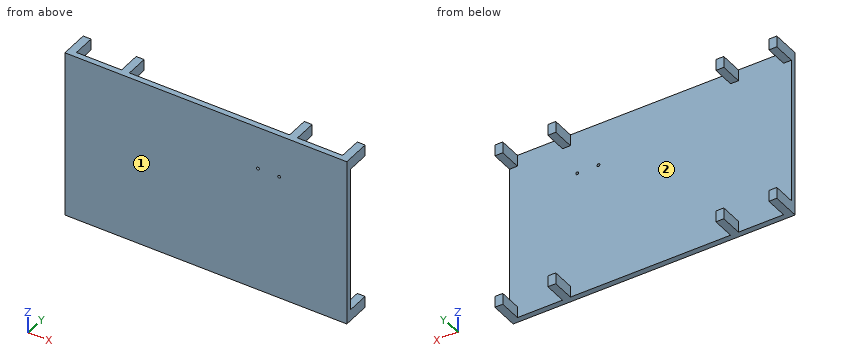
```python
from build123d import *

# Parameters (mm, degrees)
SKETCH1_W           = 250
SKETCH1_H           = 150
BOSS_EXTRUDE1_DEPTH = 5
SKETCH2_W           = 7
SKETCH2_H           = 10
BOSS_EXTRUDE2_DEPTH = 20
SKETCH3_R           = 1.25
CUT_EXTRUDE1_DEPTH  = 148.139389696


with BuildPart() as part:
    # Sketch1 → Boss-Extrude1 (new body)
    with BuildSketch(Plane(origin=(0, 0, 0), x_dir=(1, 0, 0), z_dir=(0, 1, 0))):
        Rectangle(SKETCH1_W, SKETCH1_H)
    extrude(amount=BOSS_EXTRUDE1_DEPTH)

    # Sketch2 → Boss-Extrude2 (add)
    with BuildSketch(Plane(origin=(0, 5, 0), x_dir=(1, 0, 0), z_dir=(0, 1, 0))):
        with Locations((-121.5, -70)):
            Rectangle(SKETCH2_W, SKETCH2_H)
        with Locations((-74.5, -70)):
            Rectangle(SKETCH2_W, SKETCH2_H)
        with Locations((-121.5, 70)):
            Rectangle(SKETCH2_W, SKETCH2_H)
        with Locations((-74.5, 70)):
            Rectangle(SKETCH2_W, SKETCH2_H)
        with Locations((121.5, 70)):
            Rectangle(SKETCH2_W, SKETCH2_H)
        with Locations((74.5, 70)):
            Rectangle(SKETCH2_W, SKETCH2_H)
        with Locations((121.5, -70)):
            Rectangle(SKETCH2_W, SKETCH2_H)
        with Locations((74.5, -70)):
            Rectangle(SKETCH2_W, SKETCH2_H)
    extrude(amount=BOSS_EXTRUDE2_DEPTH)

    # Sketch3 → Cut-Extrude1 (cut, through all)
    with BuildSketch(Plane(origin=(0, 5, 0), x_dir=(1, 0, 0), z_dir=(0, 1, 0))):
        with Locations(Location((46.2, -37, 0), (0, 0, 270))):
            Circle(SKETCH3_R)
        with Locations(Location((65, -37, 0), (0, 0, 270))):
            Circle(SKETCH3_R)
    extrude(amount=-CUT_EXTRUDE1_DEPTH, mode=Mode.SUBTRACT)


solid = part.part
```
Here's how the part is built. I have some questions about the finished solid (model axes, mm). Face numbers are marked on the shaded views. Round coordinates to 2 decimals unless told otherwise and drop trailing zeros. Order: outer loops, then holes, each group sorted by start corner. A loop starts at its lowest first (then second) coordinate and runs counter-clockwise, first axis right, second up. Notation, with made-up numbers: M 68,47 L 92,47 A14 cw 92,65 Z; hole C -4,29 d11. An arc over 180 degrees is marked long. One line per question, with ' | ' between items.
1) I need wall thicknesses on line 1 along X through (y, z) = (16.25, -68); line 2 along X through (y, z) = (3.7, 37); line 3 along Z through (x, y) = (65, 1.8). Which ranges of each line are inside material? Lowest first, please.
Working result:
line 1: -125 to -118, -78 to -71, 71 to 78, 118 to 125 | line 2: -125 to 44.95, 47.45 to 63.75, 66.25 to 125 | line 3: -75 to 35.75, 38.25 to 75
2) I want a section at C-C, the plane z = 57.5. Write out the boundary of the cut face in (x, y).
Working result:
outline: M -125,0 L 125,0 L 125,5 L -125,5 Z
3) I want a section at A-A, the plane y = 19.5. State how many separate pieces and enclosed holes the cut face has, then the cut area to 3 significant figures.
Working result:
separate pieces: 8 | enclosed holes: 0 | area: 560 mm²
4) I want a section at B-B, the plane x = 97.5. Write out the boundary of the cut face in (y, z), then the cut area to 3 significant figures.
Working result:
outline: M 0,-75 L 5,-75 L 5,75 L 0,75 Z | area: 750 mm²
5) If we mould it in two halves opening along X, with no side actions, what happens to the marked faces 1 and 2? For each: +X half, -X half, draft (parallel to the pull), parting line (faces both ways), or undercut.
Working result:
face 1: draft | face 2: undercut
6) For pin 1 Ø5 at (x, z) = (-84, -57.5) entering from +Y; pin 2 Ø6 at (x, z) = (53, -43) entering from -Y, each with a flat end and sliding along its axis, tell me the tip position at first contact or that it passes through.
Working result:
pin 1: y = 5 | pin 2: y = 0
